from build123d import *

# Parameters (mm, degrees)
BOSS_EXTRUDE1_DEPTH = 1.8
FILLET2_R           = 0.5


with BuildPart() as part:
    # Sketch1 → Boss-Extrude1 (new body)
    with BuildSketch(Plane(origin=(0, 0, 0), x_dir=(1, 0, 0), z_dir=(0, 1, 0))):
        with BuildLine():
            Line((0, 4.5), (0, 6.5))
            Line((0, 6.5), (6.1, 6.5))
            Line((6.1, 6.5), (6.1, 10.5))
            Line((6.1, 10.5), (10, 14.4))
            Line((10, 14.4), (10, 83.5))
            Line((10, 83.5), (16.4, 83.5))
            ThreePointArc((16.4, 83.5), (17.2719581, 81.425344658), (17.601960582, 79.199226044))
            Line((17.601960582, 79.199226044), (18.25, 49.5))
            Line((18.25, 49.5), (12, 49.5))
            Line((12, 49.5), (12, 37.18))
            add(Edge.make_bspline(
                [(12.5, 32.33), (12.5, 33.972282338), (12, 35.554764974), (12, 37.18)],
                knots=[0, 0, 0, 0, 1, 1, 1, 1], degree=3))
            Line((12.5, 32.33), (12.5, 3.07))
            ThreePointArc((12.5, 3.07), (11.600817818, 0.899182182), (9.43, 0))
            ThreePointArc((9.43, 0), (4.205660329, 1.182650422), (0, 4.5))
        make_face()
    extrude(amount=BOSS_EXTRUDE1_DEPTH)

    # Fillet2
    fillet2_edges = [part.edges().sort_by_distance(p)[0] for p in [
        (0, 0.9, -6.5),
        (6.1, 0.9, -6.5),
        (6.1, 0.9, -10.5),
        (10, 0.9, -14.4),
        (10, 0.9, -83.5),
        (18.25, 0.9, -49.5),
        (12, 0.9, -49.5),
    ]]
    fillet(fillet2_edges, radius=FILLET2_R)


solid = part.part
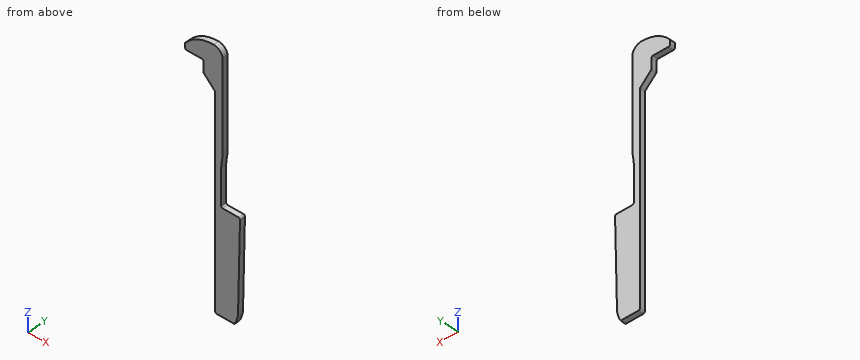
For this review, take the finished solid that the model builds, in its own axes (mm). Round coordinates to 2 decimals unless told otherwise and drop trailing zeros. Order: outer loops, then holes, each group sorted by start corner. A loop starts at its lowest first (then second) coordinate and runs counter-clockwise, first axis right, second up. Notation, with made-up numbers: M 11,-39 L 61,-39 A15 ccw 61,-34 Z; hole C 45.5,-5.5 d2. An arc over 180 degrees is marked long. Use a Markdown table: item, result. Add a question column.
Item 1: To check wall thickness, follow line 1 along Z through (x, y) = (13, 1.3); line 2 along X through (y, z) = (0.4, -6); line 3 along X through (y, z) = (1.6, -19.5). State the ranges of each line that lie inside material, in increasing order.
Item 2: Add section B-B, the plane z = -20. Give the boundary of the cut face in (x, y), then the cut area to 3 significant figures.
Item 3: Insertion check: pin 1 (0.9 mm diameter, centred on y = 1.5, z = -44.5, fed in from -X); pin 2 (0.9 mm diameter, centred on y = 0.5, z = -16.5, fed in from +X); pin 3 (0.5 mm diameter, centred on y = 0.5, z = -9, fed in from -X). Each pin has a flat end and moves straight along its axis. Give the tip position at first contact, or say it passes through.
Item 4: Add section A-A, the plane x = 15.5. Give the boundary of the cut face in (y, z).
Geometry results:
| question | item | result |
|---|---|---|
| 1 | line 1 | z = -83.5 to -49.5 |
| 1 | line 2 | x = 0 to 12.5 |
| 1 | line 3 | x = 10 to 12.5 |
| 2 | outline | M 10,0 L 12.5,0 L 12.5,1.8 L 10,1.8 Z |
| 2 | area | 4.50 mm² |
| 3 | pin 1 | stops at x = 10 |
| 3 | pin 2 | stops at x = 12.5 |
| 3 | pin 3 | stops at x = 6.1 |
| 4 | outline | M 0,-83.5 L 1.8,-83.5 L 1.8,-49.5 L 0,-49.5 Z |
